Input: part model. Units: mm. Frame: model coordinates. Face numbers are marked on the shaded views. A direction names the side the tool comes from. Give positions to 0.01 mm unless a question says otherwise; leave off trailing zeros. Loops run counter-clockwise (first coordinate to the right, second up) from the corner with the lowest first, then second, coordinate; pieces in that order, holes last. Notation, with made-up numbers: M -2,67 L 37,67 A8 cw 37,78 Z; hole C -5,64.5 d9. An arc over 180 degrees is marked long. Answer as a JSON object with one key per item and string values. Group by question number.
1) Access query for the marked faces 5, 6 and 7. Directions: +Z, -Z, +X, -X, +Y, -Y. A direction counts if a zero-diameter tool reaches every point of the face in a straight line with its end or side. Return the directions, or none.
2) Section query B-B on z = 87. Return loops of the section in (x, y).
3) Section query D-D on z = 35.5. Return loops of the section in (x, y), plus the area to 4 significant figures.
4) Ray query, L1, parallel to Z at x = 14, y = 27.5; L2, parallel to X at y = 39, z = 88; L3, parallel to Z at x = 17.75, y = 30. Return the intervals inside material, ascending.
5) Section query A-A on y = 14. Return loops of the section in (x, z).
6) Draft query along Z for the marked faces 1, 2, 3 and 4. Return one class per face: +Z half, -Z half, draft (parallel to the pull), parting line (faces both ways), or undercut.
7) First-contact query: P1, Ø10, axis at x = 9.5, z = 20, coming from the -Y side; P2, Ø5, axis at y = 21.5, z = 29.5, coming from the +X side. Flat tips, straight axial feed; report the tip coordinate or a pass-through.
8) Section query C-C on x = 13. Return loops of the section in (y, z).
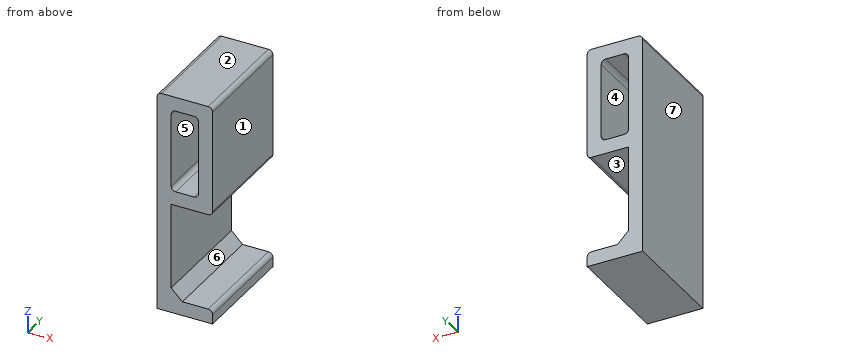
from build123d import *

# Parameters (mm, degrees)
BINDER_FACE1_W = 12.3
BINDER_FACE1_H = 37.3
PAD_DEPTH      = 50
CHAMFER_SIZE   = 5
FILLET_R       = 2
FILLET001_R    = 2
FILLET002_R    = 2
FILLET003_R    = 2
FILLET004_R    = 2
FILLET005_R    = 2
FILLET006_R    = 2
FILLET007_R    = 2


with BuildPart() as part:
    # Binder Face1 → Pad (new)
    with BuildSketch(Plane(origin=(10.393732, 0, 55.131766), x_dir=(1, 0, 0), z_dir=(0, 1, 0))):
        Polygon((14.606268, 5.131766), (-4.043732, 5.131766), (-4.043732, 48.781766), (14.606268, 48.781766), (14.606268, 55.131766), (-10.393732, 55.131766), (-10.393732, -44.868234), (14.606268, -44.868234), align=None)
        with Locations((2.106268, -19.868234)):
            Rectangle(BINDER_FACE1_W, BINDER_FACE1_H, mode=Mode.SUBTRACT)
    extrude(amount=PAD_DEPTH)

    # Chamfer
    chamfer_edges = [part.edges().sort_by_distance(p)[0] for p in [
        (6.35, 25, 6.35),
    ]]
    chamfer(chamfer_edges, length=CHAMFER_SIZE)

    # Fillet
    fillet_edges = [part.edges().sort_by_distance(p)[0] for p in [
        (25, 25, 6.35),
    ]]
    fillet(fillet_edges, radius=FILLET_R)

    # Fillet001
    fillet001_edges = [part.edges().sort_by_distance(p)[0] for p in [
        (25, 25, 50),
    ]]
    fillet(fillet001_edges, radius=FILLET001_R)

    # Fillet002
    fillet002_edges = [part.edges().sort_by_distance(p)[0] for p in [
        (25, 25, 100),
    ]]
    fillet(fillet002_edges, radius=FILLET002_R)

    # Fillet003
    fillet003_edges = [part.edges().sort_by_distance(p)[0] for p in [
        (0, 25, 100),
    ]]
    fillet(fillet003_edges, radius=FILLET003_R)

    # Fillet004
    fillet004_edges = [part.edges().sort_by_distance(p)[0] for p in [
        (6.35, 25, 93.65),
    ]]
    fillet(fillet004_edges, radius=FILLET004_R)

    # Fillet005
    fillet005_edges = [part.edges().sort_by_distance(p)[0] for p in [
        (18.65, 25, 93.65),
    ]]
    fillet(fillet005_edges, radius=FILLET005_R)

    # Fillet006
    fillet006_edges = [part.edges().sort_by_distance(p)[0] for p in [
        (6.35, 25, 56.35),
    ]]
    fillet(fillet006_edges, radius=FILLET006_R)

    # Fillet007
    fillet007_edges = [part.edges().sort_by_distance(p)[0] for p in [
        (18.65, 25, 56.35),
    ]]
    fillet(fillet007_edges, radius=FILLET007_R)


solid = part.part
Output:
{
 "1": {"face 5": "+Y, -Y", "face 6": "+X, +Y, -Y", "face 7": "+Z, -Z, -X, +Y, -Y"},
 "2": {"outline": "M 0,0 L 6.35,0 L 6.35,50 L 0,50 Z; M 18.65,0 L 25,0 L 25,50 L 18.65,50 Z"},
 "3": {"outline": "M 0,0 L 6.35,0 L 6.35,50 L 0,50 Z", "area": "317.5 mm^2"},
 "4": {"L1": "z = 0 to 6.35, 50 to 56.35, 93.65 to 100", "L2": "x = 0 to 6.35, 18.65 to 25", "L3": "z = 0 to 6.35, 50 to 56.68, 93.32 to 100"},
 "5": {"outline": "M 0,0 L 25,0 L 25,4.35 A2 ccw 23,6.35 L 11.35,6.35 L 6.35,11.35 L 6.35,50 L 23,50 A2 ccw 25,52 L 25,98 A2 ccw 23,100 L 2,100 A2 ccw 0,98 Z; hole M 6.35,58.35 A2 ccw 8.35,56.35 L 16.65,56.35 A2 ccw 18.65,58.35 L 18.65,91.65 A2 ccw 16.65,93.65 L 8.35,93.65 A2 ccw 6.35,91.65 Z"},
 "6": {"face 1": "draft", "face 2": "+Z half", "face 3": "undercut", "face 4": "undercut"},
 "7": {"P1": "stops at y = 0", "P2": "stops at x = 6.35"},
 "8": {"outline": "M 0,0 L 50,0 L 50,6.35 L 0,6.35 Z; M 0,50 L 50,50 L 50,56.35 L 0,56.35 Z; M 0,93.65 L 50,93.65 L 50,100 L 0,100 Z"}
}
